Can you work these out from the model? Positions are in its coordinate system, mm. A direction names the side the tool comes from. Give positions to 0.01 mm unless a question says otherwise; leave off trailing zeros. Write each loop counter-clockwise with the first axis right and the second up, starting at its lowest first coordinate (ties: lowest second). Pieces come first, ordered by that corner, then holes.
```python
from build123d import *

# Parameters (mm, degrees)
BOSS_EXTRUDE1_DEPTH      = 7
SKETCH2_R                = 5
CUT_EXTRUDE1_DEPTH       = 7
LPATTERN1_COUNT          = 7
LPATTERN1_PITCH          = 30
SKETCH6_R                = 5
CUT_EXTRUDE2_DEPTH       = 10
BOSS_EXTRUDE2_DEPTH      = 21
CUT_EXTRUDE3_DEPTH       = 21
CUT_EXTRUDE4_REACH       = 220.014
SKETCH9_R                = 1.5
CUT_EXTRUDE5_REACH       = 220.771
SKETCH10_W               = 5.271518542
SKETCH10_H               = 23.219312301
BOSS_EXTRUDE3_DEPTH      = 14
CUT_EXTRUDE6_DEPTH       = 1
CUT_EXTRUDE6_DEPTH_BACK  = 22
SKETCH12_W               = 22.7
SKETCH12_H               = 14.642587258
SKETCH12_H_2             = 12.3
CUT_EXTRUDE7_DEPTH       = 7
CUT_EXTRUDE7_DEPTH_BACK  = 7
SKETCH13_R               = 1
CUT_EXTRUDE8_REACH       = 184.393
SKETCH14_W               = 12
SKETCH14_H               = 12
CUT_EXTRUDE11_DEPTH      = 219.013742346
CUT_EXTRUDE11_DEPTH_BACK = 219.013742346
SKETCH16_W               = 140
SKETCH16_H               = 37.19308959
SKETCH17_W               = 7
SKETCH17_H               = 21.4
BOSS_EXTRUDE4_DEPTH      = 11.7
CUT_EXTRUDE12_REACH      = 94.641
SKETCH18_R               = 1.5
CUT_EXTRUDE13_REACH      = 95.925
SKETCH20_W               = 15.728481458
SKETCH20_H               = 11.090838969
SKETCH21_W               = 7
SKETCH21_H               = 16.279991403
CUT_EXTRUDE14_DEPTH      = 12
BOSS_EXTRUDE5_DEPTH      = 7
CUT_EXTRUDE15_DEPTH      = 116.935326799
CUT_EXTRUDE15_DEPTH_BACK = 7
SKETCH23_R               = 1.5


with BuildPart() as part:
    # Sketch1 → Boss-Extrude1 (new body)
    with BuildSketch(Plane.XY):
        with BuildLine():
            Line((-200, 0), (50, 0))
            ThreePointArc((50, 0), (65, -15), (50, -30))
            Line((50, -30), (-200, -30))
            ThreePointArc((-200, -30), (-215, -15), (-200, 0))
        make_face()
    extrude(amount=BOSS_EXTRUDE1_DEPTH)

    # Sketch2 → Cut-Extrude1 (cut)
    with BuildSketch(Plane.XY.offset(7)):
        with Locations((-185, -15)):
            Circle(SKETCH2_R)
    cut_extrude1 = extrude(amount=-CUT_EXTRUDE1_DEPTH, mode=Mode.SUBTRACT)

    # LPattern1: Cut-Extrude1 ×7
    with Locations(*[(i * LPATTERN1_PITCH, 0, 0) for i in range(1, LPATTERN1_COUNT)]):
        add(cut_extrude1, mode=Mode.SUBTRACT)

    # Sketch6 → Cut-Extrude2 (cut)
    with BuildSketch(Plane(origin=(0, 0, 0), x_dir=(-1, 0, 0), z_dir=(0, 0, -1))):
        with Locations((-50, -15)):
            Circle(SKETCH6_R)
    extrude(amount=-CUT_EXTRUDE2_DEPTH, mode=Mode.SUBTRACT)

    # Sketch7 → Boss-Extrude2 (add)
    with BuildSketch(Plane(origin=(0, 0, 0), x_dir=(0, 0, -1), z_dir=(1, 0, 0))):
        with BuildLine():
            Line((20.124409349, -8.046570755), (20.124409349, -21.391782887))
            ThreePointArc((20.124409349, -21.391782887), (10.062204675, -26.149434806), (0, -21.391782887))
            Line((0, -21.391782887), (0, -8.046570755))
            ThreePointArc((0, -8.046570755), (10.062204675, -2.930122505), (20.124409349, -8.046570755))
        make_face()
    extrude(amount=BOSS_EXTRUDE2_DEPTH)

    # Sketch8 → Cut-Extrude3 (cut)
    with BuildSketch(Plane(origin=(21, 0, 0), x_dir=(0, 0, -1), z_dir=(1, 0, 0))):
        with BuildLine():
            Line((0.343653188, -8.603738845), (0.343653188, -21.003738845))
            Line((0.343653188, -21.003738845), (3.251608919, -23.33010343))
            Line((3.251608919, -23.33010343), (6.11482687, -24.672236845))
            Line((6.11482687, -24.672236845), (10.141227113, -25.388041332))
            Line((10.141227113, -25.388041332), (14.122889575, -24.672236845))
            Line((14.122889575, -24.672236845), (17.165058648, -23.33010343))
            Line((17.165058648, -23.33010343), (19.670374355, -20.953281344))
            Line((19.670374355, -20.953281344), (19.670374355, -8.553281344))
            ThreePointArc((19.670374355, -8.553281344), (9.994377841, -3.738573545), (0.343653188, -8.603738845))
        make_face()
    extrude(amount=-CUT_EXTRUDE3_DEPTH, mode=Mode.SUBTRACT)

    # Sketch9 → Cut-Extrude4 (cut, up to next)
    with BuildSketch(Plane(origin=(0, 0, 0), x_dir=(-1, 0, 0), z_dir=(0, 0, -1)), mode=Mode.PRIVATE) as cut_extrude4_sk1:
        with Locations((-29.5, -6.25)):
            Circle(SKETCH9_R)
    cut_extrude4_tool1 = extrude(cut_extrude4_sk1.sketch, amount=-CUT_EXTRUDE4_REACH, mode=Mode.PRIVATE) & part.part
    # Sketch9 → Cut-Extrude4 (cut, up to next)
    with BuildSketch(Plane(origin=(0, 0, 0), x_dir=(-1, 0, 0), z_dir=(0, 0, -1)), mode=Mode.PRIVATE) as cut_extrude4_sk2:
        with Locations((-29.5, -23.75)):
            Circle(SKETCH9_R)
    cut_extrude4_tool2 = extrude(cut_extrude4_sk2.sketch, amount=-CUT_EXTRUDE4_REACH, mode=Mode.PRIVATE) & part.part
    add(cut_extrude4_tool1.solids().sort_by_distance((29.5, -6.25, 0))[0], mode=Mode.SUBTRACT)
    add(cut_extrude4_tool2.solids().sort_by_distance((29.5, -23.75, 0))[0], mode=Mode.SUBTRACT)

    # Cut-Extrude5: up to this face of the body (flat: up to its plane)
    cut_extrude5_end = Plane(part.part.faces().sort_by_distance((-78.33059512, -15.01080435, 0))[0])
    # Sketch10 → Cut-Extrude5 (cut, up to the picked face)
    with BuildSketch(Plane(origin=(0, 0, -20.124409349), x_dir=(-1, 0, 0), z_dir=(0, 0, -1)), mode=Mode.PRIVATE) as cut_extrude5_sk1:
        with Locations((-2.635759271, -14.539778656)):
            Rectangle(SKETCH10_W, SKETCH10_H)
    cut_extrude5_tool1 = split(extrude(cut_extrude5_sk1.sketch, amount=-CUT_EXTRUDE5_REACH, mode=Mode.PRIVATE), bisect_by=cut_extrude5_end, keep=Keep.BOTH, mode=Mode.PRIVATE)
    add(cut_extrude5_tool1.solids().sort_by(Axis((2.635759, -14.539779, -20.124409), (0, 0, 1)))[0], mode=Mode.SUBTRACT)

    # Sketch11 → Boss-Extrude3 (add)
    with BuildSketch(Plane(origin=(0, 0, 0), x_dir=(-1, 0, 0), z_dir=(0, 0, -1))):
        Polygon((60.097644306, -6.420008597), (60.097644306, -23.913431972), (36.21993437, -23.913431972), (36.21993437, -6.613282571), (31.020509523, -6.613282571), (31.020509523, -2.674883318), (65.276628567, -2.674883318), (65.276628567, -6.420008597), align=None)
        Polygon((193.975354243, -6.285954501), (193.975354243, -16.540829221), (170.097644306, -16.540829221), (170.097644306, -6.479228475), (164.898219459, -6.479228475), (164.898219459, -2.540829221), (199.154338504, -2.540829221), (199.154338504, -6.285954501), align=None)
    extrude(amount=BOSS_EXTRUDE3_DEPTH)

    # Sketch12 → Cut-Extrude6 (cut, two sides: drawn at the far end of the back side and taken through both)
    with BuildSketch(Plane(origin=(0, -2.674883318, 0), x_dir=(1, 0, 0), z_dir=(0, 1, 0)).offset(-CUT_EXTRUDE6_DEPTH_BACK)):
        with Locations((-48.226628567, 7.87504546)):
            Rectangle(SKETCH12_W, SKETCH12_H)
        with Locations((-182.104338504, 6.42306456)):
            Rectangle(SKETCH12_W, SKETCH12_H_2)
    extrude(amount=CUT_EXTRUDE6_DEPTH + CUT_EXTRUDE6_DEPTH_BACK, mode=Mode.SUBTRACT)

    # Sketch13 → Cut-Extrude7 (cut, two sides: drawn at the far end of the back side and taken through both)
    with BuildSketch(Plane(origin=(0, -2.674883318, 0), x_dir=(1, 0, 0), z_dir=(0, 1, 0)).offset(-CUT_EXTRUDE7_DEPTH_BACK)):
        with Locations(Location((-167.998219459, 8.19, 0), (0, 0, 90))):
            Circle(SKETCH13_R)
        with Locations(Location((-196.054338504, 8.19, 0), (0, 0, 90))):
            Circle(SKETCH13_R)
        with Locations(Location((-62.176628567, 8.19, 0), (0, 0, 90))):
            Circle(SKETCH13_R)
        with Locations(Location((-34.120509523, 8.19, 0), (0, 0, 90))):
            Circle(SKETCH13_R)
    extrude(amount=CUT_EXTRUDE7_DEPTH + CUT_EXTRUDE7_DEPTH_BACK, mode=Mode.SUBTRACT)

    # Cut-Extrude8: up to this face of the body (flat: up to its plane)
    cut_extrude8_end = Plane(part.part.faces().sort_by_distance((-193.975354243, -11.413391861, -7))[0])
    # Sketch14 → Cut-Extrude8 (cut, up to the picked face)
    with BuildSketch(Plane(origin=(-36.21993437, 0, 0), x_dir=(0, 0, -1), z_dir=(1, 0, 0)), mode=Mode.PRIVATE) as cut_extrude8_sk1:
        with Locations((8, -17.913431972)):
            Rectangle(SKETCH14_W, SKETCH14_H)
    cut_extrude8_tool1 = split(extrude(cut_extrude8_sk1.sketch, amount=-CUT_EXTRUDE8_REACH, mode=Mode.PRIVATE), bisect_by=cut_extrude8_end, keep=Keep.BOTH, mode=Mode.PRIVATE)
    add(cut_extrude8_tool1.solids().sort_by(Axis((-36.219934, -17.913432, -8), (-1, 0, 0)))[0], mode=Mode.SUBTRACT)

    # Sketch16 → Cut-Extrude11 (cut, two sides: drawn at the far end of the back side and taken through both)
    with BuildSketch(Plane(origin=(0, 0, 0), x_dir=(-1, 0, 0), z_dir=(0, 0, -1)).offset(-CUT_EXTRUDE11_DEPTH_BACK)):
        with Locations((145, -15.740579032)):
            Rectangle(SKETCH16_W, SKETCH16_H)
    extrude(amount=CUT_EXTRUDE11_DEPTH + CUT_EXTRUDE11_DEPTH_BACK, mode=Mode.SUBTRACT)

    # Sketch17 → Boss-Extrude4 (add)
    with BuildSketch(Plane.ZY.offset(75)):
        with Locations((3.5, -15)):
            Rectangle(SKETCH17_W, SKETCH17_H)
    extrude(amount=BOSS_EXTRUDE4_DEPTH)

    # Sketch18 → Cut-Extrude12 (cut, up to next)
    with BuildSketch(Plane(origin=(0, -4.3, 0), x_dir=(1, 0, 0), z_dir=(0, 1, 0)), mode=Mode.PRIVATE) as cut_extrude12_sk1:
        with Locations(Location((-80, -3.5, 0), (0, 0, 270))):
            Circle(SKETCH18_R)
    cut_extrude12_tool1 = extrude(cut_extrude12_sk1.sketch, amount=-CUT_EXTRUDE12_REACH, mode=Mode.PRIVATE) & part.part
    add(cut_extrude12_tool1.solids().sort_by_distance((-80, -4.3, 3.5))[0], mode=Mode.SUBTRACT)

    # Sketch20 → Cut-Extrude13 (cut, up to next)
    with BuildSketch(Plane(origin=(0, 0, 0), x_dir=(1, 0, 0), z_dir=(0, 1, 0)), mode=Mode.PRIVATE) as cut_extrude13_sk1:
        with Locations((13.135759271, 14.578989865)):
            Rectangle(SKETCH20_W, SKETCH20_H)
    cut_extrude13_tool1 = extrude(cut_extrude13_sk1.sketch, amount=-CUT_EXTRUDE13_REACH, mode=Mode.PRIVATE) & part.part
    add(cut_extrude13_tool1.solids().sort_by_distance((13.135759, 0, -14.57899))[0], mode=Mode.SUBTRACT)

    # Sketch21 → Cut-Extrude14 (cut)
    with BuildSketch(Plane.ZY.offset(86.7)):
        with Locations((3.5, -14.560004299)):
            Rectangle(SKETCH21_W, SKETCH21_H)
    extrude(amount=-CUT_EXTRUDE14_DEPTH, mode=Mode.SUBTRACT)

    # Sketch22 → Boss-Extrude5 (add)
    with BuildSketch(Plane(origin=(0, 0, 0), x_dir=(-1, 0, 0), z_dir=(0, 0, -1))):
        with BuildLine():
            ThreePointArc((-50, -20), (-55, -15), (-50, -10))
            Line((-50, -10), (-50, 0))
            Line((-50, 0), (-95, 0))
            ThreePointArc((-95, 0), (-110, -15), (-95, -30))
            Line((-95, -30), (-50, -30))
            Line((-50, -30), (-50, -20))
        make_face()
    extrude(amount=-BOSS_EXTRUDE5_DEPTH)

    # Sketch23 → Cut-Extrude15 (cut, two sides: drawn at the far end of the back side and taken through both)
    with BuildSketch(Plane.XY.offset(7).offset(-CUT_EXTRUDE15_DEPTH_BACK)):
        with Locations(Location((85.914550285, -25, 0), (0, 0, 180))):
            Circle(SKETCH23_R)
        with Locations(Location((85.914550285, -5, 0), (0, 0, 180))):
            Circle(SKETCH23_R)
    extrude(amount=CUT_EXTRUDE15_DEPTH + CUT_EXTRUDE15_DEPTH_BACK, mode=Mode.SUBTRACT)


solid = part.part
```
1) For pin 1 Ø10 at (x, z) = (-35, -1.5) entering from +Y; pin 2 Ø2 at (y, z) = (-15, 3) entering from -X; pin 3 Ø12 at (y, z) = (-10, -7) entering from +X; pin 4 Ø1.6 at (x, z) = (-48, -1) entering from -Y, each with a flat end and sliding along its axis, tell me the tip position at first contact or that it passes through.
Values follow:
pin 1: stops at y = 0
pin 2: stops at x = -74.7
pin 3: stops at x = 21
pin 4: stops at y = -23.91
2) Please list where these lines run through material, in increasing order: L1, parallel to X at y = -5.25, z = -8.19; L2, parallel to Y at x = 29.5, z = 5.75; L3, parallel to Y at x = -65.5, z = 4.5.
Values follow:
L1: x = -65.28 to -63.18, -61.18 to -59.58, -36.88 to -35.12, -33.12 to -31.02
L2: y = -30 to -25.25, -22.25 to -7.75, -4.75 to 0
L3: y = -30 to -19.97, -10.03 to 0
3) Suppose I cut it at A-A on x = 50. Write out the boundary of the cut face in (y, z).
Values follow:
outline: (-30, 0) - (-20, 0) - (-20, 7) - (-30, 7) - close; (-10, 0) - (0, 0) - (0, 7) - (-10, 7) - close
4) For faces 4 (the face through (-82, -4.3, 3)), 5 (the face through (-48, -13, -0.554)), 6 (the face through (-82, -25.7, 3)), which set-ups out of +Z, -Z, +X, -X, +Y, -Y let a thin tool reach every point of the face, with its end or its side?
Values follow:
face 4: +Z, -Z, -X, +Y
face 5: -Z, +Y, -Y
face 6: +Z, -Z, -X, -Y
5) Suppose I cut it at B-B on x = -2.5. Write out the boundary of the cut face in (y, z), plus the area to 3 significant figures.
Values follow:
outline: (-30, 0) - (-19.33, 0) - (-19.33, 7) - (-30, 7) - close; (-10.67, 0) - (0, 0) - (0, 7) - (-10.67, 7) - close
area: 149 mm2
6) If we mould it in two halves opening along X, with no side actions, what happens to faces 1 (the face through (5.272, -15.45, -0.19)), 2 (the face through (-60.098, -11, -5)), 3 (the face through (-82, -6.42, 3))? For each: +X half, -X half, draft (parallel to the pull), parting line (faces both ways), or undercut.
Values follow:
face 1: undercut
face 2: -X half
face 3: draft
